Can you work these out from the model? Positions are in its coordinate system, mm. A direction names the side the tool comes from. Give positions to 0.01 mm unless a question says otherwise; leave off trailing zeros. Loops run counter-clockwise (first coordinate to the right, second up) from the corner with the lowest first, then second, coordinate; pieces in that order, holes last. Notation, with made-up numbers: (21, -6.5) - (71, -6.5) arc R15 cw to (71, 19.5) - close; hole circle Ø11 at (55, 84.25). An arc over 180 degrees is marked (long way). Answer as a JSON object with one key per item and string values.
```python
from build123d import *

# Parameters (mm, degrees)
SKETCH3_R          = 5
CUT_EXTRUDE2_DEPTH = 107.856211799


with BuildPart() as part:
    # Sketch1 → Revolve2 (revolve)
    with BuildSketch(Plane.XY, mode=Mode.PRIVATE) as revolve2_sk:
        Polygon((-6, -5.5), (11, -5.5), (11, 5.5), (-6, 5.5), (-11, 5.5), (-33, 5.5), (-55, 5.5), (-77, 5.5), (-94, 5.5), (-94, -5.5), (-77, -5.5), (-77, -4), (-72, -4), (-72, -5.5), (-55, -5.5), (-55, -4), (-50, -4), (-50, -5.5), (-33, -5.5), (-33, -4), (-28, -4), (-28, -5.5), (-11, -5.5), (-11, -4), (-6, -4), align=None)
    revolve(revolve2_sk.sketch.rotate(Axis((-33, 5.5, 0), (-1, 0, 0)), 180), axis=Axis((-33, 5.5, 0), (-1, 0, 0)))

    # Sketch3 → Cut-Extrude2 (cut, through all)
    with BuildSketch(Plane.ZY.offset(94)):
        with Locations(Location((0, 5.5, 0), (0, 0, 270))):
            Circle(SKETCH3_R)
    extrude(amount=-CUT_EXTRUDE2_DEPTH, mode=Mode.SUBTRACT)


solid = part.part
```
1) Imagine slicing it at B-B on x = -54. Write out the boundary of the cut face in (y, z).
Check sheet entries:
{"outline": "circle Ø19 at (5.5, 0); hole circle Ø10 at (5.5, 0)"}
2) I'm going to push flat-ended pins straight in: P1, Ø2, axis at x = -60, z = 6, coming from the -Y side; P2, Ø1, axis at x = -70.5, z = 6.5, coming from the +Y side; P3, Ø10, axis at x = -3, y = 10.5, coming from the +Z side; P4, Ø1, axis at x = -3, y = -1, coming from the -Z side. Where does each tip first touch, or does it pass through?
Check sheet entries:
{"P1": "y = -4.3", "P2": "y = 14.72", "P3": "z = 11", "P4": "z = -9.22"}
3) I need wall thicknesses on L1, parallel to X at y = 9, z = -10; L2, parallel to Z at x = -66.5, y = 5.5; L3, parallel to Z at x = -53, y = 5.5. Which ranges of each line are inside material? Lowest first, please.
Check sheet entries:
{"L1": "-94 to -77, -72 to -55, -50 to -33, -28 to -11, -6 to 11", "L2": "-11 to -5, 5 to 11", "L3": "-9.5 to -5, 5 to 9.5"}
4) If we mould it in two halves opening along Z, with no side actions, what happens to faces 3 (the flat face through (-11, -3, 5)), 4 (the cylindrical face through (-63.381, 10.576, 9.759)), 5 (the cylindrical face through (-42.24, 0.73, 1.5))? For each: released by +Z, released by -Z, zero draft, split by the parting line, or undercut.
Check sheet entries:
{"face 3": "zero draft", "face 4": "split by the parting line", "face 5": "undercut"}
5) Imagine slicing it at A-A on x = -4. Write out the boundary of the cut face in (y, z).
Check sheet entries:
{"outline": "circle Ø22 at (5.5, 0); hole circle Ø10 at (5.5, 0)"}
6) Which directions (+Z, -Z, +X, -X, +Y, -Y) give clear straight access to the entire face, cutting with the end or side of a thin tool? Please do faces 1 (the cylindrical face through (-85.381, 10.576, 9.759)), 2 (the cylindrical face through (-52, -4, 0)).
Check sheet entries:
{"face 1": "+X, -X", "face 2": "none"}
